Read the model definition and answer for the solid it produces. Units are mm, in the model's axes. Face numbers are marked on the shaded views. A direction names the side the tool comes from. Give positions to 0.01 mm unless a question says otherwise; leave off trailing zeros. Order: outer loops, then holes, each group sorted by start corner. A loop starts at its lowest first (then second) coordinate and runs counter-clockwise, first axis right, second up. Notation, with made-up numbers: (71, 15.25) -> (113, 15.25) arc R20 ccw to (113, 20.25) -> close; hole circle Ø4 at (31, 10.25). An arc over 180 degrees is marked (long way). Answer as CSV lines item,"result". Start each with the question number.
1) Find section C-C (x = 63). Determine the outline of the cut face in (y, z).
2) The mould has two halves that part along Y. Classify the marked faces 3, 4 and 5: +Y half, -Y half, draft (parallel to the pull), parting line (faces both ways), or undercut.
3) Find section A-A (y = 35). Determine the outline of the cut face in (x, z), and give its area (3 significant figures).
4) Find section B-B (x = 44). Determine the outline of the cut face in (y, z).
5) Straight lines are drawn through the part: L1, parallel to Z at x = 44, y = 81.45; L2, parallel to Y at x = 5, z = 33; L3, parallel to Y at x = 40.5, z = 7. For each, find the intervals that lie inside material, in ascending order. Write a range as from..to.
6) Flat-ended cylindrical pins translate along their axes: pin 1 Ø1.9 at (x, y) = (67, 1) entering from -Z; pin 2 Ø1.5 at (x, y) = (29, 61) entering from -Z. Find the tip coordinate at first contact, or state that the pin passes through.
7) For the marked faces 1 and 2, determine the directions among +Z, -Z, +X, -X, +Y, -Y from which every point of the face is accessible in a straight line to the end or side of a thin tool.
8) Find section D-D (z = 12.5). State how many separate pieces and enclosed holes the cut face has, and give its area (3 significant figures).
```python
from build123d import *

# Parameters (mm, degrees)
CYLINDER006_R            = 1.45
CYLINDER006_DEPTH        = 46.5
ARRAY003_X_COUNT         = 2
ARRAY003_X_PITCH         = 58
ARRAY003_Y_COUNT         = 2
ARRAY003_Y_PITCH         = 69
CYLINDER005_R            = 6
CYLINDER005_DEPTH        = 44.5
ARRAY002_X_COUNT         = 2
ARRAY002_X_PITCH         = 58
ARRAY002_Y_COUNT         = 2
ARRAY002_Y_PITCH         = 69
CYLINDER004_R            = 2.2
CYLINDER004_DEPTH        = 10
ARRAY001_X_COUNT         = 2
ARRAY001_X_PITCH         = 20
ARRAY001_Y_COUNT         = 2
ARRAY001_Y_PITCH         = 20
ARRAY001_PLACEMENT_ANGLE = 90
BOX020_W                 = 12
BOX020_H                 = 30
BOX020_DEPTH             = 8
BOX006_W                 = 68
BOX006_H                 = 79
BOX006_DEPTH             = 46.5
BOX005_W                 = 70
BOX005_H                 = 83
BOX005_DEPTH             = 47.5


with BuildPart() as screw_hole_array:
    # Cylinder006 → Cylinder006 (new body)
    with BuildSketch(Plane(origin=(5, 5, 0), x_dir=(1, 0, 0), z_dir=(0, 0, 1))):
        Circle(CYLINDER006_R)
    extrude(amount=CYLINDER006_DEPTH)

    # Array003 X: screw hole array ×2


with BuildPart() as screw_hole_array_1:
    add(screw_hole_array.part)
    with Locations(*[(i * ARRAY003_X_PITCH, 0, 0) for i in range(1, ARRAY003_X_COUNT)]):
        add(screw_hole_array.part)

    # Array003 Y: screw hole array ×2


with BuildPart() as screw_hole_array_2:
    add(screw_hole_array_1.part)
    with Locations(*[(0, i * ARRAY003_Y_PITCH, 0) for i in range(1, ARRAY003_Y_COUNT)]):
        add(screw_hole_array_1.part)


with BuildPart() as bolt_stand_fusion:
    # Cylinder005 → Cylinder005 (new body)
    with BuildSketch(Plane(origin=(5, 5, 2.5), x_dir=(1, 0, 0), z_dir=(0, 0, 1))):
        Circle(CYLINDER005_R)
    extrude(amount=CYLINDER005_DEPTH)

    # Array002 X: bolt stand fusion ×2


with BuildPart() as bolt_stand_fusion_1:
    add(bolt_stand_fusion.part)
    with Locations(*[(i * ARRAY002_X_PITCH, 0, 0) for i in range(1, ARRAY002_X_COUNT)]):
        add(bolt_stand_fusion.part)

    # Array002 Y: bolt stand fusion ×2


with BuildPart() as bolt_stand_fusion_2:
    add(bolt_stand_fusion_1.part)
    with Locations(*[(0, i * ARRAY002_Y_PITCH, 0) for i in range(1, ARRAY002_Y_COUNT)]):
        add(bolt_stand_fusion_1.part)

    # Cut001004: cut screw hole array
    add(screw_hole_array_2.part, mode=Mode.SUBTRACT)


with BuildPart() as top_insert_hole_array:
    # Cylinder004 → Cylinder004 (new body)
    with BuildSketch(Plane.XY):
        Circle(CYLINDER004_R)
    extrude(amount=CYLINDER004_DEPTH)

    # Array001 X: top insert hole array ×2


with BuildPart() as top_insert_hole_array_1:
    add(top_insert_hole_array.part)
    with Locations(*[(i * ARRAY001_X_PITCH, 0, 0) for i in range(1, ARRAY001_X_COUNT)]):
        add(top_insert_hole_array.part)

    # Array001 Y: top insert hole array ×2


with BuildPart() as top_insert_hole_array_2:
    add(top_insert_hole_array_1.part)
    with Locations(*[(0, i * ARRAY001_Y_PITCH, 0) for i in range(1, ARRAY001_Y_COUNT)]):
        add(top_insert_hole_array_1.part)


with BuildPart() as top_insert_hole_array_3:
    # Array001 placement: moved
    add(top_insert_hole_array_2.part.moved(Location((24, 88, 16))).rotate(Axis((24, 88, 16), (1, 0, 0)), ARRAY001_PLACEMENT_ANGLE))


with BuildPart() as micro_usb_hole:
    # Box020 → Box020 (new body)
    with BuildSketch(Plane(origin=(-15, 30.2, 23.65), x_dir=(0, 0, 1), z_dir=(0, 1, 0))):
        with Locations((6, 15)):
            Rectangle(BOX020_W, BOX020_H)
    extrude(amount=BOX020_DEPTH)


with BuildPart() as back_box_extract_fusion:
    # Box006 → Box006 (new body)
    with BuildSketch(Plane.XY):
        with Locations((34, 39.5)):
            Rectangle(BOX006_W, BOX006_H)
    extrude(amount=BOX006_DEPTH)

    # Fusion006: union top insert hole array, micro usb hole
    add(top_insert_hole_array_3.part)
    add(micro_usb_hole.part)


with BuildPart() as back_box_fusion:
    # Box005 → Box005 (new body)
    with BuildSketch(Plane(origin=(-1, -1, 0), x_dir=(1, 0, 0), z_dir=(0, 0, 1))):
        with Locations((35, 41.5)):
            Rectangle(BOX005_W, BOX005_H)
    extrude(amount=BOX005_DEPTH)

    # Cut001003: cut back box extract fusion
    add(back_box_extract_fusion.part, mode=Mode.SUBTRACT)

    # Fusion007: union bolt stand fusion
    add(bolt_stand_fusion_2.part)


solid = back_box_fusion.part
```
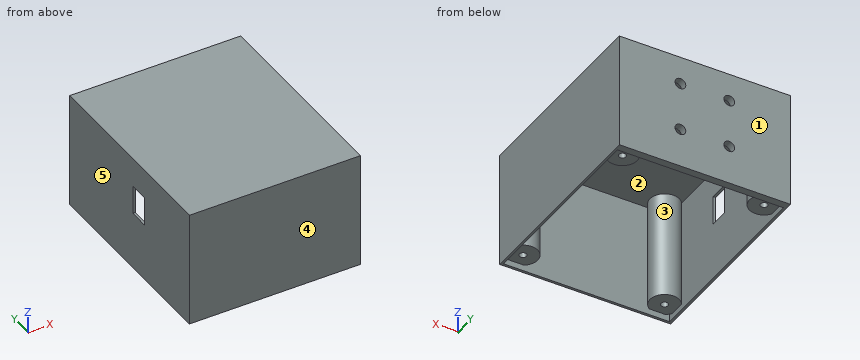
Findings below:
1,outline,"(-1, 0) -> (0, 0) -> (0, 2.5) -> (3.55, 2.5) -> (3.55, 46.5) -> (6.45, 46.5) -> (6.45, 2.5) -> (11, 2.5) -> (11, 46.5) -> (68, 46.5) -> (68, 2.5) -> (72.55, 2.5) -> (72.55, 46.5) -> (75.45, 46.5) -> (75.45, 2.5) -> (79, 2.5) -> (79, 0) -> (82, 0) -> (82, 47.5) -> (-1, 47.5) -> close"
2,face 3,"undercut"
2,face 4,"-Y half"
2,face 5,"draft"
3,outline,"(-1, 0) -> (0, 0) -> (0, 23.65) -> (-1, 23.65) -> close; (-1, 35.65) -> (0, 35.65) -> (0, 46.5) -> (68, 46.5) -> (68, 0) -> (69, 0) -> (69, 47.5) -> (-1, 47.5) -> close"
3,area,"151 mm²"
4,outline,"(-1, 0) -> (0, 0) -> (0, 46.5) -> (79, 46.5) -> (79, 38.2) -> (82, 38.2) -> (82, 47.5) -> (-1, 47.5) -> close; (79, 0) -> (82, 0) -> (82, 13.8) -> (79, 13.8) -> close; (79, 18.2) -> (82, 18.2) -> (82, 33.8) -> (79, 33.8) -> close"
5,L1,"0..13.8, 18.2..33.8, 38.2..47.5"
5,L2,"-1..3.55, 6.45..11, 68..72.55, 75.45..82"
5,L3,"-1..0, 79..82"
6,pin 1,"z = 2.5"
6,pin 2,"z = 46.5"
7,face 1,"+Z, -Z, +X, -X, +Y"
7,face 2,"-Z"
8,separate pieces,"1"
8,enclosed holes,"9"
8,area,"828 mm²"
